Autodesk Inventor part; units mm, degrees
ref_plane "YZ Plane" through (0, 0, 0) normal (1, 0, 0) x (0, 1, 0)
ref_plane "XZ Plane" through (0, 0, 0) normal (0, 1, 0) x (-1, 0, 0)
ref_plane "XY Plane" through (0, 0, 0) normal (0, 0, 1) x (1, 0, 0)
sketch "Sketch1" plane through (0, 0, 0) normal (0, 1, 0) x (-1, 0, 0)
  circle A0 centre (0, 0) radius 4.75
  dimension "d0" = 9.5
extrude "Extrusion1" add sketch "Sketch1" along normal blind 45
sketch "Sketch2" plane through (0, 45, 0) normal (0, 1, 0) x (1, 0, 0)
  circle A0 centre (0, 0) radius 10
  dimension "d3" = 20
extrude "Extrusion2" add sketch "Sketch2" along normal blind 5
fillet "Fillet1" radius 4 1 edges at (4.75, 0, 0)
fillet "Fillet2" radius 4 1 edges at (-10, 50, 0)
equation "\"BendRadius\" = Thickness"
equation "\"BendReliefWidth\" = Thickness"
equation "\"BendReliefDepth\" = 0.5 * Thickness"
equation "\"CornerReliefSize\" = 4 * Thickness"
equation "\"MinimumRemnant\" = 2 * Thickness"
equation "\"TransitionRadius\" = BendRadius"
equation "\"JacobiRadiusSize\" = BendRadius"
equation "\"GapSize\" = Thickness"
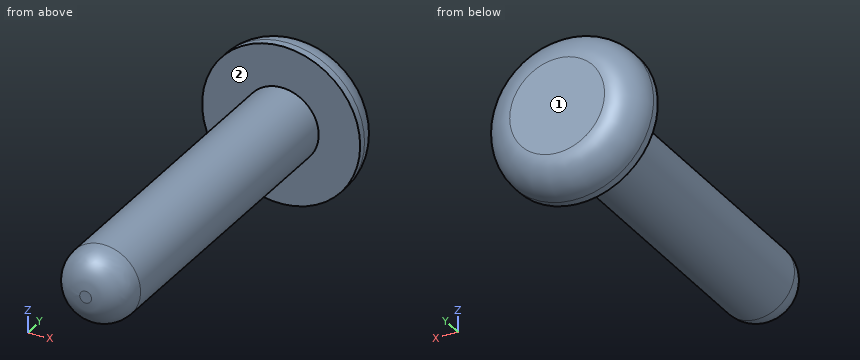
The model under review builds one solid part; all positions refer to its coordinate system, in mm. Face numbers are marked on the shaded views. A direction names the side the tool comes from. Round coordinates to 2 decimals unless told otherwise and drop trailing zeros. Write each loop counter-clockwise with the first axis right and the second up, starting at its lowest first coordinate (ties: lowest second). Pieces come first, ordered by that corner, then holes. Notation, with made-up numbers: M 20.25,39 L 63.25,39 A13 cw 63.25,64 Z; hole C 86.5,82.5 d5. An arc over 180 degrees is marked long. Use a Markdown table: item, result. Add a question column.
Q1. Machinability: for the marked faces 1 and 2, which of the approach directions +Z, -Z, +X, -X, +Y, -Y give a long, thin tool a straight path to every point of the face, cutting with its end or side? Answer none if there is none.
Q2. Insertion check: pin 1 (6 mm diameter, centred on x = 1.5, z = -4.5, fed in from -Y); pin 2 (10 mm diameter, centred on x = 4, z = 6.5, fed in from -Y); pin 3 (5 mm diameter, centred on y = 18, z = 6.5, fed in from -X). Each pin has a flat end and moves straight along its axis. Give the tip position at first contact, or say it passes through.
Q3. We need section A-A, the plane y = 16.5. State the section outline as (x, z) points, plus the area to 3 significant figures.
Q4. We need section B-B, the plane y = 46.5. State the section outline as (x, z) points, plus the area to 3 significant figures.
Q5. To check wall thickness, follow line 1 (Y direction, x = 6, z = 1); line 2 (Z direction, x = -0.25, y = 10.5); line 3 (Y direction, x = 0, z = -1). State the ranges of each line that lie inside material, in increasing order.
Findings below:
| question | item | result |
|---|---|---|
| 1 | face 1 | +Z, -Z, +X, -X, +Y |
| 1 | face 2 | -Y |
| 2 | pin 1 | stops at y = 0.13 |
| 2 | pin 2 | stops at y = 0.47 |
| 2 | pin 3 | stops at x = -2.56 |
| 3 | outline | C 0,0 d9.5 |
| 3 | area | 70.9 mm² |
| 4 | outline | C 0,0 d19.94 |
| 4 | area | 312 mm² |
| 5 | line 1 | y = 45 to 50 |
| 5 | line 2 | z = -4.74 to 4.74 |
| 5 | line 3 | y = 0.01 to 50 |
